Check sheet for the modelled part. Datum: model origin and axes. Units: mm. A direction names the side the tool comes from. Give positions to 0.01 mm unless a question says otherwise; leave off trailing zeros. Order: outer loops, then holes, each group sorted by start corner. A loop starts at its lowest first (then second) coordinate and runs counter-clockwise, first axis right, second up.
```python
from build123d import *

# Parameters (mm, degrees)
BOSS_EXTRUDE1_DEPTH  = 2
BOSS_EXTRUDE6_DEPTH  = 4.5
CUT_EXTRUDE6_DEPTH   = 4.5
BOSS_EXTRUDE14_DEPTH = 2.3
SKETCH32_R           = 3
CUT_EXTRUDE7_DEPTH   = 2.3
SKETCH33_W           = 22.343119157
SKETCH33_H           = 2
SKETCH33_W_2         = 17.499973406
SKETCH33_H_2         = 1.5
BOSS_EXTRUDE15_DEPTH = 1.2
SKETCH35_W           = 5.479645996
SKETCH35_H           = 3.871139505
CUT_EXTRUDE8_DEPTH   = 2.4
SKETCH36_W           = 3.7
SKETCH36_H           = 1.871139505
CUT_EXTRUDE9_DEPTH   = 4.4
SKETCH37_R           = 3.9
BOSS_EXTRUDE16_DEPTH = 4.4
CUT_EXTRUDE10_DEPTH  = 7.4
SKETCH43_R           = 2.5
BOSS_EXTRUDE17_DEPTH = 1.2
SKETCH44_R           = 0.95
CUT_EXTRUDE11_DEPTH  = 11
SKETCH45_R           = 2
CUT_EXTRUDE12_DEPTH  = 4.5
SKETCH49_R           = 0.75
CUT_EXTRUDE13_DEPTH  = 3
SKETCH51_W           = 3
SKETCH51_H           = 3.965585241
CUT_EXTRUDE14_DEPTH  = 6.8
FILLET1_R            = 1.5
FILLET3_R            = 1


with BuildPart() as part:
    # Sketch3 → Boss-Extrude1 (new body)
    with BuildSketch(Plane.XY):
        with BuildLine():
            Line((8, 0), (9, -2.543145751))
            Line((9, -2.543145751), (9, -7.043145751))
            Line((9, -7.043145751), (26.499973406, -7.043145751))
            Line((26.499973406, -7.043145751), (30.050225938, -4.992893219))
            ThreePointArc((30.050225938, -4.992893219), (41.467130134, -2.721929777), (34.999973406, 6.956854249))
            Line((34.999973406, 6.956854249), (31.999973406, 7.456854249))
            Line((31.999973406, 7.456854249), (5.656854249, 7.456854249))
            Line((5.656854249, 7.456854249), (5.656854249, 5.656854249))
            ThreePointArc((5.656854249, 5.656854249), (7.39103626, 3.061467459), (8, 0))
        make_face()
    extrude(amount=BOSS_EXTRUDE1_DEPTH)

    # Sketch22 → Boss-Extrude6 (add)
    with BuildSketch(Plane.XY.offset(2)):
        with BuildLine():
            Line((5.656854249, 7.456854249), (26.499973406, 7.456854249))
            Line((26.499973406, 7.456854249), (31.999973406, 7.456854249))
            Line((31.999973406, 7.456854249), (31.999973406, 2.128860495))
            Line((31.999973406, 2.128860495), (28.275099672, 2.128860495))
            Line((28.275099672, 2.128860495), (28.275099672, -6.018019485))
            Line((28.275099672, -6.018019485), (26.499973406, -7.043145751))
            Line((26.499973406, -7.043145751), (9, -7.043145751))
            Line((9, -7.043145751), (9, -2.543145751))
            Line((9, -2.543145751), (8, 0))
            ThreePointArc((8, 0), (7.39103626, 3.061467459), (5.656854249, 5.656854249))
            Line((5.656854249, 5.656854249), (5.656854249, 7.456854249))
        make_face()
    extrude(amount=BOSS_EXTRUDE6_DEPTH)

    # Sketch26 → Cut-Extrude6 (cut)
    with BuildSketch(Plane.XY.offset(2)):
        Polygon((18.098080448, 5.3), (2.530052458, 5.3), (2.530052458, 4), (18.098080448, 4), (31.999973406, 4), (31.999973406, 5.3), align=None)
    extrude(amount=CUT_EXTRUDE6_DEPTH, mode=Mode.SUBTRACT)


with BuildPart() as body_2:
    # Sketch31 → Boss-Extrude14 (new body)
    with BuildSketch(Plane.XY.offset(6.5)):
        with BuildLine():
            Line((2.432688066, 5.656854249), (0, 5.656854249))
            ThreePointArc((0, 5.656854249), (-5.656854249, 0), (0, -5.656854249))
            Line((0, -5.656854249), (9, -5.656854249))
            Line((9, -5.656854249), (9, -7.043145751))
            Line((9, -7.043145751), (9, -8.543145751))
            Line((9, -8.543145751), (26.499973406, -8.543145751))
            Line((26.499973406, -8.543145751), (26.499973406, -7.043145751))
            Line((26.499973406, -7.043145751), (26.499973406, 2.128860495))
            Line((26.499973406, 2.128860495), (28.275099672, 2.128860495))
            Line((28.275099672, 2.128860495), (31.999973406, 2.128860495))
            Line((31.999973406, 2.128860495), (31.999973406, 7.456854249))
            Line((31.999973406, 7.456854249), (31.999973406, 8.956854249))
            Line((31.999973406, 8.956854249), (5.656854249, 8.956854249))
            Line((5.656854249, 8.956854249), (5.656854249, 7.456854249))
            Line((5.656854249, 7.456854249), (5.656854249, 5.656854249))
            Line((5.656854249, 5.656854249), (2.432688066, 5.656854249))
        make_face()
    extrude(amount=BOSS_EXTRUDE14_DEPTH)

    # Sketch32 → Cut-Extrude7 (cut)
    with BuildSketch(Plane.XY.offset(8.8)):
        Circle(SKETCH32_R)
    extrude(amount=-CUT_EXTRUDE7_DEPTH, mode=Mode.SUBTRACT)

    # Sketch33 → Boss-Extrude15 (add)
    with BuildSketch(Plane.XY.offset(8.8)):
        with Locations((16.828413828, 7.956854249)):
            Rectangle(SKETCH33_W, SKETCH33_H)
        with Locations((17.749986703, -7.793145751)):
            Rectangle(SKETCH33_W_2, SKETCH33_H_2)
        with BuildLine():
            Line((7, -4.156854249), (25.499973406, -4.156854249))
            Line((25.499973406, -4.156854249), (25.499973406, -2.156854249))
            Line((25.499973406, -2.156854249), (7, -2.156854249))
            ThreePointArc((7, -2.156854249), (6, -3.156854249), (7, -4.156854249))
        make_face()
        with BuildLine():
            Line((25.499973406, 2.172006245), (7, 2.172006245))
            ThreePointArc((7, 2.172006245), (6, 3.172006245), (7, 4.172006245))
            Line((7, 4.172006245), (25.499973406, 4.172006245))
            Line((25.499973406, 4.172006245), (25.499973406, 2.172006245))
        make_face()
    extrude(amount=BOSS_EXTRUDE15_DEPTH)


with BuildPart() as cut_extrude8_tool:
    # Sketch35 → Cut-Extrude8 (new body)
    with BuildSketch(Plane.XY.offset(8.8)):
        with Locations((29.260150408, 4.064430247)):
            Rectangle(SKETCH35_W, SKETCH35_H)
    extrude(amount=-CUT_EXTRUDE8_DEPTH)


with BuildPart() as part_1:
    add(part.part)

    # Cut-Extrude8: cut by cut_extrude8_tool
    add(cut_extrude8_tool.part, mode=Mode.SUBTRACT)

    # Sketch36 → Cut-Extrude9 (cut)
    with BuildSketch(Plane.XY.offset(6.4)):
        with Locations((30.149973406, 3.064430247)):
            Rectangle(SKETCH36_W, SKETCH36_H)
    extrude(amount=-CUT_EXTRUDE9_DEPTH, mode=Mode.SUBTRACT)

    # Sketch37 → Boss-Extrude16 (add)
    with BuildSketch(Plane.XY.offset(2)):
        with Locations((34.999973406, -0.043145751)):
            Circle(SKETCH37_R)
    extrude(amount=BOSS_EXTRUDE16_DEPTH)

    # Sketch39 → Cut-Extrude10 (cut, through all)
    with BuildSketch(Plane.XY.offset(6.4)):
        with BuildLine():
            Line((33.999973406, 0.936650147), (33.999973406, -1.022941648))
            ThreePointArc((33.999973406, -1.022941648), (36.399973406, -0.043145751), (33.999973406, 0.936650147))
        make_face()
    extrude(amount=-CUT_EXTRUDE10_DEPTH, mode=Mode.SUBTRACT)


with BuildPart() as body_2_1:
    add(body_2.part)

    # Cut-Extrude8: cut by cut_extrude8_tool
    add(cut_extrude8_tool.part, mode=Mode.SUBTRACT)

    # Sketch43 → Boss-Extrude17 (add)
    with BuildSketch(Plane.XY.offset(8.8)):
        with Locations((16.5, 0)):
            Circle(SKETCH43_R)
        with Locations((23, 0)):
            Circle(SKETCH43_R)
    extrude(amount=BOSS_EXTRUDE17_DEPTH)


with BuildPart() as cut_extrude11_tool:
    # Sketch44 → Cut-Extrude11 (new body, through all)
    with BuildSketch(Plane.XY.offset(10)):
        with Locations((16.5, 0)):
            Circle(SKETCH44_R)
        with Locations((23, 0)):
            Circle(SKETCH44_R)
    extrude(amount=-CUT_EXTRUDE11_DEPTH)


with BuildPart() as part_2:
    add(part_1.part)

    # Cut-Extrude11: cut by cut_extrude11_tool
    add(cut_extrude11_tool.part, mode=Mode.SUBTRACT)

    # Sketch45 → Cut-Extrude12 (cut)
    with BuildSketch(Plane(origin=(0, 0, 0), x_dir=(-1, 0, 0), z_dir=(0, 0, -1))):
        with Locations((-16.5, 0)):
            Circle(SKETCH45_R)
        with Locations((-23, 0)):
            Circle(SKETCH45_R)
    extrude(amount=-CUT_EXTRUDE12_DEPTH, mode=Mode.SUBTRACT)


with BuildPart() as body_2_2:
    add(body_2_1.part)

    # Cut-Extrude11: cut by cut_extrude11_tool
    add(cut_extrude11_tool.part, mode=Mode.SUBTRACT)

    # Sketch49 → Cut-Extrude13 (cut)
    with BuildSketch(Plane.XZ.offset(-6.956854249)):
        with Locations((24.999973406, 10)):
            Circle(SKETCH49_R)
    extrude(amount=-CUT_EXTRUDE13_DEPTH, mode=Mode.SUBTRACT)


with BuildPart() as cut_extrude14_tool:
    # Sketch51 → Cut-Extrude14 (new body)
    with BuildSketch(Plane.XY.offset(8.8)):
        with Locations((30.499973406, 6.974061629)):
            Rectangle(SKETCH51_W, SKETCH51_H)
    extrude(amount=-CUT_EXTRUDE14_DEPTH)


with BuildPart() as part_3:
    add(part_2.part)

    # Cut-Extrude14: cut by cut_extrude14_tool
    add(cut_extrude14_tool.part, mode=Mode.SUBTRACT)

    # Fillet3
    fillet3_edges = [part_3.edges().sort_by_distance(p)[0] for p in [
        (28.275099672, -6.018019485, 4.25),
        (28.999973406, 7.456854249, 4.25),
        (9, -7.043145751, 3.25),
        (5.656854249, 7.456854249, 3.25),
        (17.749986703, -7.043145751, 0),
        (18.828413828, 7.456854249, 0),
    ]]
    fillet(fillet3_edges, radius=FILLET3_R)


with BuildPart() as body_2_3:
    add(body_2_2.part)

    # Cut-Extrude14: cut by cut_extrude14_tool
    add(cut_extrude14_tool.part, mode=Mode.SUBTRACT)

    # Fillet1
    fillet1_edges = [body_2_3.edges().sort_by_distance(p)[0] for p in [
        (17.328413828, 8.956854249, 6.5),
        (17.749986703, -8.543145751, 6.5),
    ]]
    fillet(fillet1_edges, radius=FILLET1_R)


solid = part_3.part
```
Q1. Material ranges on line 1 (Y direction, x = 23, z = 2.6); line 2 (Y direction, x = 26.5, z = 6.25); line 3 (Y direction, x = 23, z = 5.3), recorded low to high.
Q2. Sectioned sample at B-B, the plane x = 23. Record the cut outline in (y, z), plus the area to 3 significant figures.
Q3. Sectioned sample at D-D, the plane x = 36. Record the cut outline in (y, z), plus the area to 3 significant figures.
Q4. Sectioned sample at A-A, the plane z = 5.5. Count the separate pieces of the cut face and the enclosed holes in it, plus the area to 3 significant figures.
Q5. Tool access check on faces 4 (the flat face through (17, 4, 4)), 5 (the flat face through (27.51, -6.46, 2.48)), 6 (the flat face through (37, 0, 6.4)), 7 (the cylindrical face through (28.7, 7.17, 4.22)), 8 (the cylindrical face through (18.1, -1.2, 2.2)). Record the directions out of +Z, -Z, +X, -X, +Y, -Y that give a thin tool (end or side, any length) a straight path to the whole face; none if there is none.
Q6. Draft check along Y on faces 1 (the flat face through (28.3, 3, 4)), 2 (the flat face through (31, 1, 2)), 3 (the cylindrical face through (38.6, -1.54, 4.17)). Enter one of: pulls with the +Y half, pulls with the -Y half, needs draft (parallel to the pull), parting line crosses it, or undercut.
Q7. Go/stop test with flat-tipped pins: P1, Ø1, axis at y = -4.5, z = 5, coming from the -X side; P2, Ø0.8, axis at x = 28.5, y = 5.5, coming from the +Z side; P3, Ø3, axis at y = 3.5, z = 3, coming from the +X side. Record where each tip stops, or that it passes through.
Filled in:
1. line 1: y = -7.04 to -2, 2 to 4, 5.3 to 7.46
1. line 2: y = -7.04 to 4, 5.3 to 7.46
1. line 3: y = -7.04 to -0.95, 0.95 to 4, 5.3 to 7.46
2. outline: (-7.04, 1) arc R1 ccw to (-6.04, 0) - (-2, 0) - (-2, 4.5) - (-0.95, 4.5) - (-0.95, 6.5) - (-7.04, 6.5) - close; (0.95, 4.5) - (2, 4.5) - (2, 0) - (6.46, 0) arc R1 ccw to (7.46, 1) - (7.46, 6.5) - (5.3, 6.5) - (5.3, 2) - (4, 2) - (4, 6.5) - (0.95, 6.5) - close
2. area: 66.2 mm2
3. outline: (-6.97, 0) - (-1.02, 0) - (-1.02, 6.4) - (-3.81, 6.4) - (-3.81, 2) - (-6.97, 2) - close; (0.94, 0) - (6.46, 0) arc R1 ccw to (6.89, 0.1) - (6.89, 2) - (3.73, 2) - (3.73, 6.4) - (0.94, 6.4) - close
3. area: 48.3 mm2
4. separate pieces: 3
4. enclosed holes: 3
4. area: 305 mm2
5. face 4: +Z, +X, -X
5. face 5: +Z, -Z, -Y
5. face 6: +Z, +X, +Y, -Y
5. face 7: +Z, +X, +Y
5. face 8: -Z
6. face 1: needs draft
6. face 2: undercut
6. face 3: parting line crosses it
7. P1: stops at x = 9
7. P2: stops at z = 6.4
7. P3: stops at x = 41.57
